from build123d import *

# Parameters (mm, degrees)
F1_DEPTH      = 30
F2_R          = 4.25
F3_DEPTH      = 41.001
F3_DEPTH_BACK = 41.001


with BuildPart() as f1:
    # F0 (on Top) → F1 (new body)
    with BuildSketch(Plane.XY):
        Polygon((11, 30), (11, 0), (15, 0), (15, 26), (41, 26), (41, 30), align=None)
        Polygon((-11, 30), (11, 30), (41, 30), (41, 32), (-41, 32), (-41, 30), align=None)
        Polygon((-11, 0), (-11, 30), (-41, 30), (-41, 26), (-15, 26), (-15, 0), align=None)
    extrude(amount=F1_DEPTH)

    # F2 (on Right) → F3 (cut, two sides)
    with BuildSketch(Plane.YZ) as f3_sk:
        with Locations((12.5, 15.5769230769)):
            Circle(F2_R)
    extrude(amount=-F3_DEPTH, mode=Mode.SUBTRACT)
    extrude(f3_sk.sketch, amount=F3_DEPTH_BACK, mode=Mode.SUBTRACT)


solid = f1.part
Check sheet for the modelled part. Datum: model origin and axes. Units: mm. A direction names the side the tool comes from. Round coordinates to 2 decimals unless told otherwise and drop trailing zeros. Write each loop counter-clockwise with the first axis right and the second up, starting at its lowest first coordinate (ties: lowest second). Pieces come first, ordered by that corner, then holes. Notation, with made-up numbers: (-12.75, -26) -> (17.25, -26) arc R14 cw to (17.25, -6) -> close; hole circle Ø1 at (82, 70.5). An arc over 180 degrees is marked (long way). Answer as CSV lines item,"result". Start each with the question number.
1) Tool access check on faces 4 (the flat face through (-11, 15, 11)), 5 (the flat face through (-15, 16, 11)), 6 (the flat face through (28, 26, 15)). Record the directions out of +Z, -Z, +X, -X, +Y, -Y that give a thin tool (end or side, any length) a straight path to the whole face; none if there is none.
2) Go/stop test with flat-tipped pins: P1, Ø9, axis at y = 20, z = 12, coming from the -X side; P2, Ø13, axis at x = -31.5, z = 21, coming from the -Y side; P3, Ø7.5, axis at y = 12.5, z = 15.58, coming from the -X side; P4, Ø13, axis at y = 19, z = 18, coming from the +X side. Record where each tip stops, or that it passes through.
3) Section check D-D on z = 7.5. Enter the section's corners in (x, y).
4) Material ranges on line 1 (X direction, y = 22, z = 7); line 2 (Z direction, x = 13.15, y = 12.5); line 3 (X direction, y = 28.5, z = 20.75), recorded low to high. Write a range as from..to.
5) Release check for a two-part mould opening along Y. For faces 1 (the flat face through (-13, 0, 15)), 2 (the cylindrical face through (12.97, 11.95, 19.79)), 3 (the flat face through (1, 32, 15)) record: pulls with the +Y half, pulls with the -Y half, needs draft (parallel to the pull), parting line crosses it, or undercut.
6) Section check A-A on y = 12.5. Enter the section's corners in (x, z).
7) Section check C-C on z = 16.5. Enter the section's corners in (x, y).
8) Section check B-B on y = 6. Enter the section's corners in (x, z).
Found:
1,face 4,"+Z, -Z, -Y"
1,face 5,"+Z, -Z, -X, -Y"
1,face 6,"+Z, -Z, +X, -Y"
2,P1,"stops at x = -15"
2,P2,"stops at y = 26"
2,P3,"passes through"
2,P4,"stops at x = 15"
3,outline,"(-41, 26) -> (-15, 26) -> (-15, 0) -> (-11, 0) -> (-11, 30) -> (11, 30) -> (11, 0) -> (15, 0) -> (15, 26) -> (41, 26) -> (41, 32) -> (-41, 32) -> close"
4,line 1,"x = -15..-11, 11..15"
4,line 2,"z = 0..11.33, 19.83..30"
4,line 3,"x = -41..-11, 11..41"
5,face 1,"pulls with the -Y half"
5,face 2,"undercut"
5,face 3,"pulls with the +Y half"
6,outline,"(-15, 0) -> (-11, 0) -> (-11, 11.33) -> (-15, 11.33) -> close; (-15, 19.83) -> (-11, 19.83) -> (-11, 30) -> (-15, 30) -> close; (11, 0) -> (15, 0) -> (15, 11.33) -> (11, 11.33) -> close; (11, 19.83) -> (15, 19.83) -> (15, 30) -> (11, 30) -> close"
7,outline,"(-41, 26) -> (-15, 26) -> (-15, 16.65) -> (-11, 16.65) -> (-11, 30) -> (11, 30) -> (11, 16.65) -> (15, 16.65) -> (15, 26) -> (41, 26) -> (41, 32) -> (-41, 32) -> close; (-15, 0) -> (-11, 0) -> (-11, 8.35) -> (-15, 8.35) -> close; (11, 0) -> (15, 0) -> (15, 8.35) -> (11, 8.35) -> close"
8,outline,"(-15, 0) -> (-11, 0) -> (-11, 30) -> (-15, 30) -> close; (11, 0) -> (15, 0) -> (15, 30) -> (11, 30) -> close"
